Verification items for the finished model (mm, model axes). Face numbers are marked on the shaded views. A direction names the side the tool comes from. Round coordinates to 2 decimals unless told otherwise and drop trailing zeros. Loops run counter-clockwise (first coordinate to the right, second up) from the corner with the lowest first, then second, coordinate; pieces in that order, holes last. Notation, with made-up numbers: M 38,68.25 L 64,68.25 A12 ccw 64,77.25 Z; hole C -2.75,-25 d4. An arc over 180 degrees is marked long. Answer as CSV lines item,"result".
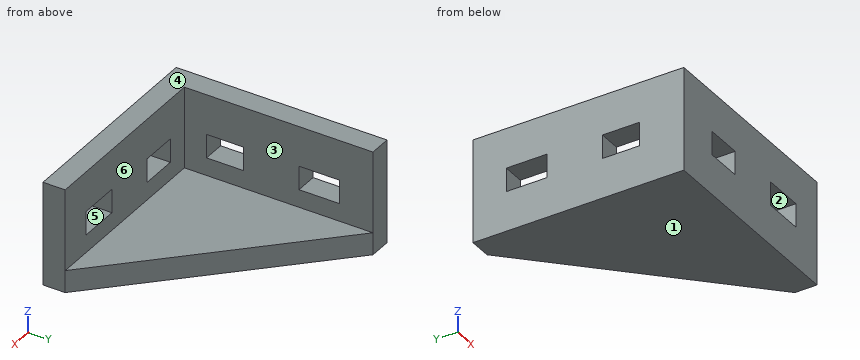
```python
from build123d import *

# Parameters (mm, degrees)
F1_DEPTH = 14
F2_W     = 10
F2_H     = 6.4
F2_W_2   = 11
F3_DEPTH = 25
F5_DEPTH = 6
F6_W     = 10
F6_H     = 6.4
F6_W_2   = 11
F7_DEPTH = 25


with BuildPart() as f1:
    # F0 (on Top) → F1 (new body, symmetric)
    with BuildSketch(Plane.XY):
        Polygon((6, 57), (0, 57), (0, 0), (57, 0), (57, 6), (6, 6), align=None)
    extrude(amount=F1_DEPTH, both=True)

    # F2 (on face) → F3 (cut)
    with BuildSketch(Plane(origin=(0, 0, 0), x_dir=(0, -1, 0), z_dir=(-1, 0, 0))):
        with Locations((-17, 0)):
            Rectangle(F2_W, F2_H)
        with Locations((-42.5, 0)):
            Rectangle(F2_W_2, F2_H)
    extrude(amount=-F3_DEPTH, mode=Mode.SUBTRACT)

    # F4 (on face) → F5 (join)
    with BuildSketch(Plane(origin=(0, 0, -14), x_dir=(1, 0, 0), z_dir=(0, 0, -1))):
        Polygon((6, -57), (57, -6), (6, -6), align=None)
    extrude(amount=-F5_DEPTH)

    # F6 (on face) → F7 (cut)
    with BuildSketch(Plane.XZ):
        with Locations((17, 0)):
            Rectangle(F6_W, F6_H)
        with Locations((42.5, 0)):
            Rectangle(F6_W_2, F6_H)
    extrude(amount=-F7_DEPTH, mode=Mode.SUBTRACT)


solid = f1.part
```
1) Material ranges on probe 1 along Y at (x, z) = (5, -1.75); probe 2 along X at (y, z) = (51.5, -2.5), recorded low to high.
Here are the results:
probe 1,"y = 0 to 12, 22 to 37, 48 to 57"
probe 2,"x = 0 to 6"
2) Section check A-A (y = 43). Record the cut outline in (x, z).
Here are the results:
outline,"M 0,-14 L 20,-14 L 20,-8 L 6,-8 L 6,-3.2 L 0,-3.2 Z; M 0,3.2 L 6,3.2 L 6,14 L 0,14 Z"
3) Section check D-D (x = 25.5). Record the cut outline in (y, z), plus the area to 3 significant figures.
Here are the results:
outline,"M 0,-14 L 37.5,-14 L 37.5,-8 L 6,-8 L 6,14 L 0,14 Z"
area,"357 mm^2"
4) Draft check along X on the marked faces 1, 2 and 3. Enter one of: +X half, -X half, draft (parallel to the pull), parting line (faces both ways), or undercut.
Here are the results:
face 1,"draft"
face 2,"undercut"
face 3,"+X half"
5) Set-up check for the marked faces 4, 5 and 6: record each of +Z, -Z, +X, -X, +Y, -Y from which the full face is reachable in a straight line by a thin tool's end or side.
Here are the results:
face 4,"+Z, +X, -X, +Y, -Y"
face 5,"+Y, -Y"
face 6,"+Z, +X, +Y"
6) Section check B-B (z = 2.25). Record the cut outline in (x, y), plus the area to 3 significant figures.
Here are the results:
outline,"M 0,0 L 12,0 L 12,6 L 6,6 L 6,12 L 0,12 Z; M 0,22 L 6,22 L 6,37 L 0,37 Z; M 0,48 L 6,48 L 6,57 L 0,57 Z; M 22,0 L 37,0 L 37,6 L 22,6 Z; M 48,0 L 57,0 L 57,6 L 48,6 Z"
area,"396 mm^2"
7) Go/stop test with flat-tipped pins: pin 1 (8 mm diameter, centred on x = 41, z = 2.5, fed in from +Y); pin 2 (1.5 mm diameter, centred on y = 13.5, z = 5.5, fed in from +X); pin 3 (10 mm diameter, centred on x = 21.5, y = 18, fed in from +Z). Record where each tip stops, or that it passes through.
Here are the results:
pin 1,"stops at y = 6"
pin 2,"stops at x = 6"
pin 3,"stops at z = -8"
8) Section check C-C (x = 46.5). Record the cut outline in (y, z), plus the area to 3 significant figures.
Here are the results:
outline,"M 0,-14 L 16.5,-14 L 16.5,-8 L 6,-8 L 6,-3.2 L 0,-3.2 Z; M 0,3.2 L 6,3.2 L 6,14 L 0,14 Z"
area,"193 mm^2"
